Input: part model. Units: mm. Frame: model coordinates. Face numbers are marked on the shaded views. Coordinates: 2 decimals unless noted, no trailing zeros. Loops run counter-clockwise (first coordinate to the right, second up) from the corner with the lowest first, then second, coordinate; pieces in that order, holes last. Notation, with made-up numbers: (44.25, 73) -> (95.25, 73) arc R12 ccw to (95.25, 85) -> close; hole circle Ø8 at (10, 5). An arc over 180 degrees is marked (long way). Put each result on its own line as item: value. Start each with the question number.
1) Cut plane A-A (x = 12.7). Return the cut outline in (y, z), plus the area to 3 significant figures.
2) Material intervals for L1, parallel to Y at x = 12.7, z = 19.5; L2, parallel to Y at x = 65, z = 23.5; L3, parallel to X at y = 65.5, z = 11.75, sorted ascending.
3) Cut plane C-C (z = 18.25). State how many separate pieces and enclosed holes the cut face has, plus the area to 3 significant figures.
4) Pull-direction query (Y, two-part tool) for the marked faces 1, 2 and 3; classes: pulls with the +Y half, pulls with the -Y half, needs draft (parallel to the pull), parting line crosses it, or undercut.
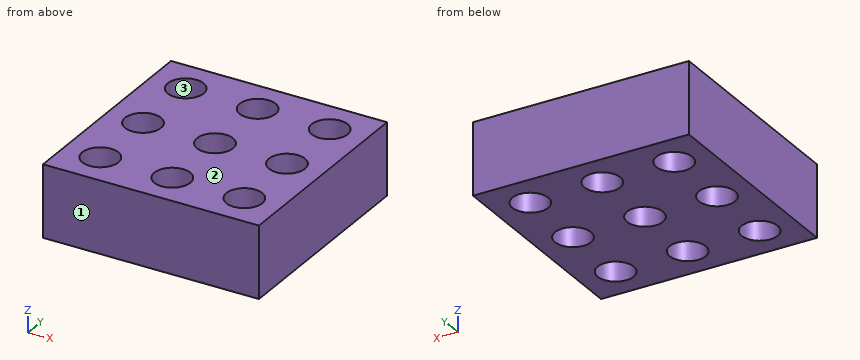
from build123d import *

# Parameters (mm, degrees)
SKETCH2_W            = 76.2
SKETCH2_H            = 76.2
BOSS_EXTRUDE1_DEPTH  = 25.4
SKETCH3_R            = 6.35
CUT_EXTRUDE1_DEPTH   = 111.716033166
LPATTERN1_COUNT      = 3
LPATTERN1_PITCH      = 25.4
LPATTERN1_COUNT_DIR2 = 3
LPATTERN1_PITCH_DIR2 = 25.4


with BuildPart() as part:
    # Sketch2 → Boss-Extrude1 (new body)
    with BuildSketch(Plane.XY):
        with Locations((38.1, 38.1)):
            Rectangle(SKETCH2_W, SKETCH2_H)
    extrude(amount=BOSS_EXTRUDE1_DEPTH)

    # Sketch3 → Cut-Extrude1 (cut, through all)
    with BuildSketch(Plane.XY.offset(25.4)):
        with Locations((12.7, 12.7)):
            Circle(SKETCH3_R)
    cut_extrude1 = extrude(amount=-CUT_EXTRUDE1_DEPTH, mode=Mode.SUBTRACT)

    # LPattern1: Cut-Extrude1 3 × 3
    with Locations(*[(j * LPATTERN1_PITCH_DIR2, i * LPATTERN1_PITCH, 0) for i in range(LPATTERN1_COUNT) for j in range(LPATTERN1_COUNT_DIR2) if (i, j) != (0, 0)]):
        add(cut_extrude1, mode=Mode.SUBTRACT)


solid = part.part
Results found:
1. outline: (0, 0) -> (6.35, 0) -> (6.35, 25.4) -> (0, 25.4) -> close; (19.05, 0) -> (31.75, 0) -> (31.75, 25.4) -> (19.05, 25.4) -> close; (44.45, 0) -> (57.15, 0) -> (57.15, 25.4) -> (44.45, 25.4) -> close; (69.85, 0) -> (76.2, 0) -> (76.2, 25.4) -> (69.85, 25.4) -> close
1. area: 968 mm2
2. L1: y = 0 to 6.35, 19.05 to 31.75, 44.45 to 57.15, 69.85 to 76.2
2. L2: y = 0 to 6.53, 18.87 to 31.93, 44.27 to 57.33, 69.67 to 76.2
2. L3: x = 0 to 6.67, 18.73 to 32.07, 44.13 to 57.47, 69.53 to 76.2
3. separate pieces: 1
3. enclosed holes: 9
3. area: 4,670 mm2
4. face 1: pulls with the -Y half
4. face 2: needs draft
4. face 3: undercut
